from build123d import *

# Parameters (mm, degrees)
SZKIC2_R                    = 80
DODANIE_WYCI_GNI_CIE2_DEPTH = 200
ZAOKR_GLENIE1_R             = 60
WYTNIJ_WYCI_GNI_CIE1_DEPTH  = 135


with BuildPart() as part:
    # Szkic2 → Dodanie-wyciągnięcie2 (new body)
    with BuildSketch(Plane(origin=(0, 0, 0), x_dir=(1, 0, 0), z_dir=(0, 1, 0))):
        Circle(SZKIC2_R)
    extrude(amount=DODANIE_WYCI_GNI_CIE2_DEPTH)

    # Zaokrąglenie1
    zaokr_glenie1_edges = [part.edges().sort_by_distance(p)[0] for p in [
        (-80, 200, 0),
    ]]
    fillet(zaokr_glenie1_edges, radius=ZAOKR_GLENIE1_R)

    # Szkic5 → Wytnij-wyciągnięcie1 (cut)
    with BuildSketch(Plane(origin=(0, 200, 0), x_dir=(1, 0, 0), z_dir=(0, 1, 0))):
        Polygon((46.75, 0), (46.75, 80.000117874), (-48.25, 80.000117874), (-48.25, 0), (-48.25, -80.000327), (46.75, -80.000327), align=None)
    extrude(amount=-WYTNIJ_WYCI_GNI_CIE1_DEPTH, mode=Mode.SUBTRACT)


solid = part.part
Can you work these out from the model? Positions are in its coordinate system, mm. Give positions to 0.01 mm unless a question says otherwise; leave off trailing zeros. Write each loop counter-clockwise with the first axis right and the second up, starting at its lowest first coordinate (ties: lowest second). Pieces come first, ordered by that corner, then holes. Notation, with made-up numbers: M 22.5,22.25 L 66.5,22.25 A25 cw 66.5,36.25 Z; hole C 57,-5 d11. An arc over 180 degrees is marked long. Answer in a Markdown table with one row per item. Add a question column.
Item 1: For pin 1 Ø4 at (x, z) = (18.5, 42.5) entering from +Y; pin 2 Ø2 at (x, y) = (-54.5, 45) entering from +Z; pin 3 Ø6 at (x, y) = (42.5, 62.5) entering from +Z; pin 4 Ø4 at (x, z) = (-27, 24.5) entering from -Y, each with a flat end and sliding along its axis, tell me the tip position at first contact or that it passes through.
Item 2: Imagine slicing it at A-A, the plane x = 0. Write out the boundary of the cut face in (y, z).
Item 3: Please list where these lines run through material, in increasing order: L1, parallel to Y at x = 7.5, z = 40.5; L2, parallel to X at y = 112.5, z = -56.5; L3, parallel to X at y = 157, z = 4.5.
Item 4: Imagine slicing it at B-B, the plane y = 15.5. Write out the boundary of the cut face in (x, z).
Item 5: We'd pull the mould along X, two halves only. Please class faces 1 (the flat face through (-1, 65, -1)), 2 (the cylindrical face through (-79.923, 53.464, -3.517)), 3 (the flat face through (-1, 0, -1)): released by +X, released by -X, zero draft, split by the parting line, or undercut.
Item 6: Imagine slicing it at C-C, the plane x = 33. Write out the boundary of the cut face in (y, z), plus the area to 3 significant figures.
Evaluation:
| question | item | result |
|---|---|---|
| 1 | pin 1 | stops at y = 65 |
| 1 | pin 2 | stops at z = 59.48 |
| 1 | pin 3 | stops at z = 69.57 |
| 1 | pin 4 | stops at y = 0 |
| 2 | outline | M 0,-80 L 65,-80 L 65,80 L 0,80 Z |
| 3 | L1 | y = 0 to 65 |
| 3 | L2 | x = -56.64 to -48.25, 46.75 to 56.64 |
| 3 | L3 | x = -77.41 to -48.25, 46.75 to 77.41 |
| 4 | outline | C 0,0 d160 |
| 5 | face 1 | undercut |
| 5 | face 2 | split by the parting line |
| 5 | face 3 | zero draft |
| 6 | outline | M 0,-72.88 L 65,-72.88 L 65,72.88 L 0,72.88 Z |
| 6 | area | 9,470 mm² |
